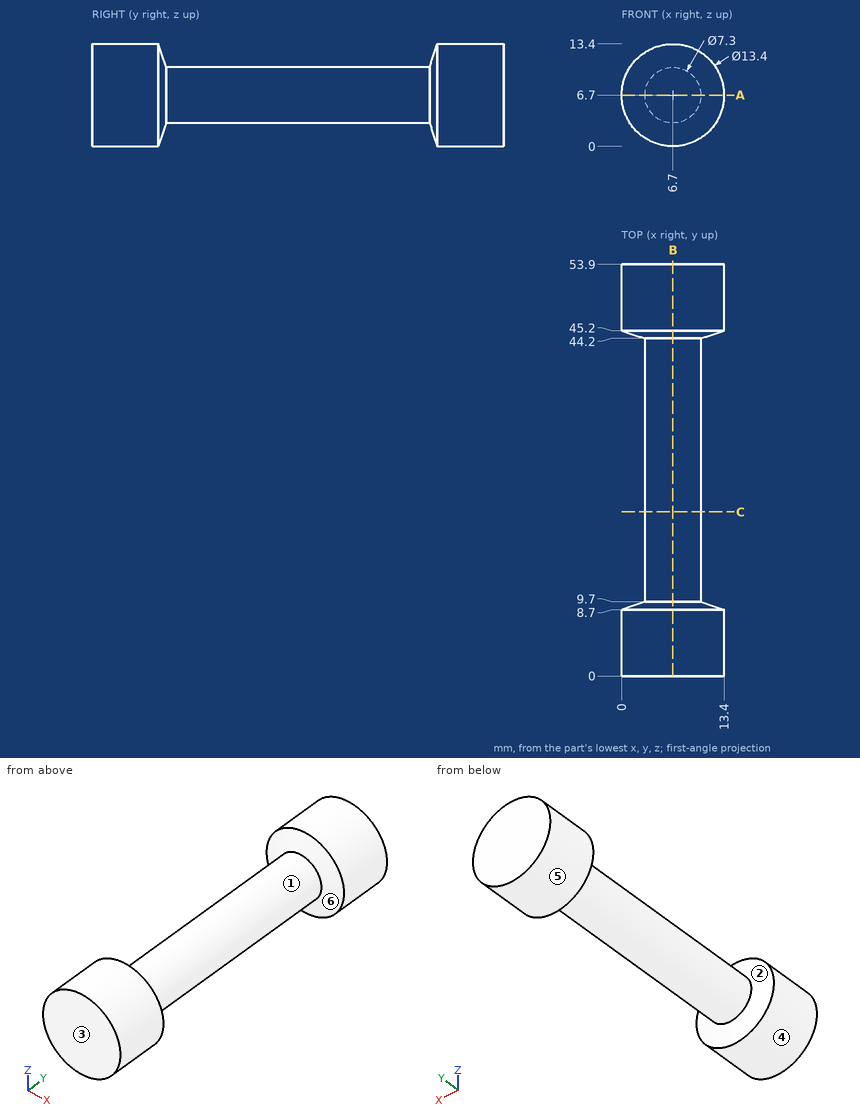
For this review, use the dimensioned drawing (mm, ordinates from the lowest corner) and the shaded views. A direction names the side the tool comes from. Round coordinates to 2 decimals unless told otherwise and drop trailing zeros. Write each loop counter-clockwise with the first axis right and the second up, starting at its lowest first coordinate (ties: lowest second). Pieces come first, ordered by that corner, then holes. Notation, with made-up numbers: (31, 45.25) -> (71, 45.25) arc R20 ccw to (71, 56.25) -> close; hole circle Ø2 at (-35.5, 44.5). An arc over 180 degrees is marked (long way). Answer in a Markdown table with one row per item.
Q1. For the marked faces 5 and 6, list the 3-axis set-ups (+Z, -Z, +X, -X, +Y, -Y) from which the entire face can be reached by the end or side of a thin tool; tool diameter is ignored.
The answers:
| item | result |
|---|---|
| face 5 | +Y, -Y |
| face 6 | none |
Q2. Take a section at A-A, the plane z = 6.7. State the section outline as (x, y) points.
The answers:
| item | result |
|---|---|
| outline | (0, 0) -> (13.4, 0) -> (13.4, 8.7) -> (10.35, 9.7) -> (10.35, 44.2) -> (13.4, 45.2) -> (13.4, 53.9) -> (0, 53.9) -> (0, 45.2) -> (3.05, 44.2) -> (3.05, 9.7) -> (0, 8.7) -> close |
Q3. To check wall thickness, follow L1, parallel to Z at x = 6.5, y = 29; L2, parallel to Y at x = 11.5, z = 6; L3, parallel to Y at x = 8.25, z = 12. State the ranges of each line that lie inside material, in increasing order. Write a range as [from, to].
The answers:
| item | result |
|---|---|
| L1 | [3.06, 10.34] |
| L2 | [0, 9.31], [44.59, 53.9] |
| L3 | [0, 9.09], [44.81, 53.9] |
Q4. Draft analysis for pull direction Y (two halves, no side actions). For the marked faces 1, 2, 3 and 4, state which applies: +Y half, -Y half, draft (parallel to the pull), parting line (faces both ways), or undercut.
The answers:
| item | result |
|---|---|
| face 1 | undercut |
| face 2 | undercut |
| face 3 | -Y half |
| face 4 | draft |
Q5. Take a section at B-B, the plane x = 6.7. State the section outline as (y, z) points, then the cut area to 3 significant figures.
The answers:
| item | result |
|---|---|
| outline | (0, 0) -> (8.7, 0) -> (9.7, 3.05) -> (44.2, 3.05) -> (45.2, 0) -> (53.9, 0) -> (53.9, 13.4) -> (45.2, 13.4) -> (44.2, 10.35) -> (9.7, 10.35) -> (8.7, 13.4) -> (0, 13.4) -> close |
| area | 506 mm² |
Q6. Take a section at C-C, the plane y = 21.5. State the section outline as (x, z) points, then the cut area to 3 significant figures.
The answers:
| item | result |
|---|---|
| outline | circle Ø7.3 at (6.7, 6.7) |
| area | 41.9 mm² |
Q7. Clearance check with flat-ended pins moving along their axes: pin 1 Ø5 at (x, y) = (6, 39.5) entering from +Z; pin 2 Ø2 at (x, y) = (3, 8.5) entering from -Z; pin 3 Ø4 at (x, y) = (11.5, 31) entering from +Z. State where each tip first meets the part, or that it passes through.
The answers:
| item | result |
|---|---|
| pin 1 | z = 10.35 |
| pin 2 | z = 0.57 |
| pin 3 | z = 9.04 |
